```python
from build123d import *

# Parameters (mm, degrees)
SKETCH_1_W          = 180
SKETCH_1_H          = 50
EXTRUDE_1_DEPTH     = 30
SKETCH_2_W          = 40
SKETCH_2_H          = 50
EXTRUDE_2_DEPTH     = 80
FILLET_1_R          = 25
SKETCH_3_R          = 12.5
CUT_EXTRUDE_2_DEPTH = 145.913767462
SKETCH_7_W          = 25
SKETCH_7_H          = 50
EXTRUDE_5_DEPTH     = 80
EXTRUDE_6_REACH     = 213.019
SKETCH_9_W          = 25.5
SKETCH_9_H          = 50
CUT_EXTRUDE_3_DEPTH = 401.320460854
SKETCH_10_W         = 65
SKETCH_10_H         = 50
EXTRUDE_7_DEPTH     = 80
SKETCH_11_W         = 50
SKETCH_11_H         = 30
EXTRUDE_8_DEPTH     = 10
SKETCH_12_W         = 50
SKETCH_12_H         = 30
CUT_EXTRUDE_4_DEPTH = 5
SKETCH_13_R         = 7.5
CUT_EXTRUDE_5_DEPTH = 412.96204223


with BuildPart() as part:
    # Sketch 1 → Extrude 1 (new body)
    with BuildSketch(Plane(origin=(0, 0, 0), x_dir=(1, 0, 0), z_dir=(0, 1, 0))):
        with Locations((90, -25)):
            Rectangle(SKETCH_1_W, SKETCH_1_H)
    extrude(amount=EXTRUDE_1_DEPTH)

    # Sketch 2 → Extrude 2 (add)
    with BuildSketch(Plane.XZ):
        with Locations((90, 25)):
            Rectangle(SKETCH_2_W, SKETCH_2_H)
    extrude(amount=EXTRUDE_2_DEPTH)

    # Fillet 1
    fillet_1_edges = [part.edges().sort_by_distance(p)[0] for p in [
        (90, -80, 50),
        (90, -80, 0),
    ]]
    fillet(fillet_1_edges, radius=FILLET_1_R - 0.0001)  # a hair under: the kernel refuses the full size

    # Sketch 3 → Cut-Extrude 2 (cut, through all)
    with BuildSketch(Plane(origin=(110, 0, 0), x_dir=(0, 0, -1), z_dir=(1, 0, 0))):
        with Locations((-25, -55)):
            Circle(SKETCH_3_R)
    extrude(amount=-CUT_EXTRUDE_2_DEPTH, mode=Mode.SUBTRACT)

    # Sketch 7 → Extrude 5 (add)
    with BuildSketch(Plane(origin=(0, 30, 0), x_dir=(1, 0, 0), z_dir=(0, 1, 0))):
        with Locations((19.5, -25)):
            Rectangle(SKETCH_7_W, SKETCH_7_H)
        with Locations((160.5, -25)):
            Rectangle(SKETCH_7_W, SKETCH_7_H)
    extrude(amount=EXTRUDE_5_DEPTH)

    # Extrude 6: up to this face of the body (flat: up to its plane)
    extrude_6_end = Plane(part.part.faces().sort_by_distance((7, 70, 25))[0])
    # Sketch 8 → Extrude 6 (add, up to the picked face)
    with BuildSketch(Plane(origin=(173, 0, 0), x_dir=(0, 0, -1), z_dir=(1, 0, 0)), mode=Mode.PRIVATE) as extrude_6_sk1:
        with BuildLine():
            Line((0, 110), (-79.29372145, 110))
            add(Edge.make_bspline(
                [(-79.29372145, 110), (123.322725029, 174.375095478), (335.808448859, 110)],
                knots=[0, 0, 0, 1, 1, 1], degree=2))
            add(Edge.make_bspline(
                [(335.808448859, 110), (344.655163531, 85.008885119), (332.386652106, 65.024574676)],
                knots=[0, 0, 0, 1, 1, 1], degree=2))
            add(Edge.make_bspline(
                [(332.386652106, 65.024574676), (334.882025134, 94.793074398), (307.328252939, 102.88474179)],
                knots=[0, 0, 0, 1, 1, 1], degree=2))
            add(Edge.make_bspline(
                [(307.328252939, 102.88474179), (153.571097441, 138.708355764), (0, 110)],
                knots=[0, 0, 0, 1, 1, 1], degree=2))
        make_face()
    extrude_6_tool1 = split(extrude(extrude_6_sk1.sketch, amount=-EXTRUDE_6_REACH, mode=Mode.PRIVATE), bisect_by=extrude_6_end, keep=Keep.BOTH, mode=Mode.PRIVATE)
    add(extrude_6_tool1.solids().sort_by(Axis((173, 122.914419, -143.709252), (-1, 0, 0)))[0])

    # Sketch 9 → Cut-Extrude 3 (cut, through all)
    with BuildSketch(Plane(origin=(0, 30, 0), x_dir=(1, 0, 0), z_dir=(0, 1, 0))):
        Polygon((57.5, -50), (32, -50), (32, 0), (57.5, 0), (57.5, 350.332715619), (7, 350.332715619), (7, -79.29372145), (57.5, -79.29372145), align=None)
        Polygon((148, -50), (122.5, -50), (122.5, -79.29372145), (173, -79.29372145), (173, 350.332715619), (122.5, 350.332715619), (122.5, 0), (148, 0), align=None)
        with Locations((44.75, -25)):
            Rectangle(SKETCH_9_W, SKETCH_9_H)
        with Locations((135.25, -25)):
            Rectangle(SKETCH_9_W, SKETCH_9_H)
    extrude(amount=CUT_EXTRUDE_3_DEPTH, mode=Mode.SUBTRACT)


with BuildPart() as cut_extrude_3_piece_1:
    # of the separate pieces the step leaves, piece 1, a body of its own (cut_extrude_3_pieces)
    add(part.part.solids().sort_by_distance((122.5, 110, 0))[0])



with BuildPart() as cut_extrude_3_piece_2:
    # of the separate pieces the step leaves, piece 2, a body of its own (cut_extrude_3_pieces)
    add(part.part.solids().sort_by_distance((110, -55.0001, 0))[0])


with BuildPart() as cut_extrude_3_piece_1_1:
    add(cut_extrude_3_piece_1.part)

    add(cut_extrude_3_piece_2.part)  # Extrude 7 merges Cut-Extrude 3 piece 2
    # Sketch 10 → Extrude 7 (add)
    with BuildSketch(Plane.XZ.offset(-110)):
        with Locations((90, 25)):
            Rectangle(SKETCH_10_W, SKETCH_10_H)
    extrude(amount=EXTRUDE_7_DEPTH)

    # Sketch 11 → Extrude 8 (add)
    with BuildSketch(Plane.ZY):
        with Locations((25, 15)):
            Rectangle(SKETCH_11_W, SKETCH_11_H)
    extrude(amount=EXTRUDE_8_DEPTH)

    # Sketch 12 → Cut-Extrude 4 (cut)
    with BuildSketch(Plane.ZY.offset(10)):
        with Locations((25, 15)):
            Rectangle(SKETCH_12_W, SKETCH_12_H)
    extrude(amount=-CUT_EXTRUDE_4_DEPTH, mode=Mode.SUBTRACT)

    # Sketch 13 → Cut-Extrude 5 (cut, through all)
    with BuildSketch(Plane.ZY.offset(5)):
        with Locations((25, 15)):
            Circle(SKETCH_13_R)
    extrude(amount=-CUT_EXTRUDE_5_DEPTH, mode=Mode.SUBTRACT)


solid = cut_extrude_3_piece_1_1.part
```
CAD build for the part. Positions are in the model's coordinates, mm. A direction names the side the tool comes from. Round coordinates to 2 decimals unless told otherwise and drop trailing zeros. Order: outer loops, then holes, each group sorted by start corner. A loop starts at its lowest first (then second) coordinate and runs counter-clockwise, first axis right, second up.
Item 1: Mould opens along Z. For faces 5 (the face through (151, 30, 25)), 6 (the face through (89, 26, 0)), 7 (the face through (89, 26, 50)) say: pulls with the +Z half, pulls with the -Z half, needs draft (parallel to the pull), parting line crosses it, or undercut.
Item 2: Saw through at C-C on y = -62. Write the cut outline in (x, z).
Item 3: Pin check, flat tip, straight feed: pin 1 (8 mm diameter, centred on x = 56.5, y = 35, fed in from +Z). Stop position of the tip, or through.
Item 4: Tool access for faces 1 (the face through (27, 30, 25)), 2 (the face through (122.5, 124, -85)), 3 (the face through (70, -31, 25)), 4 (the face through (145, 0, 25)): list every direction of +Z, -Z, +X, -X, +Y, -Y with a clear straight run to the whole face (end or side of a thin tool).
Item 5: Saw through at B-B on x = 6.5. Write the cut outline in (y, z).
Item 6: Probe line 1 along Y through (x, z) = (100.5, 25); line 2 along Y through (x, z) = (48, 25); line 3 along Z through (x, y) = (143, 18). List the from-to ranges inside material, lowest first.
Item 7: Saw through at A-A on y = 15. Write the cut outline in (x, z), then the cut area to 4 significant figures.
Item 8: Saw through at D-D on y = -35.5. Write the cut outline in (x, z), then the cut area to 3 significant figures.
Reported:
1. face 5: needs draft
1. face 6: undercut
1. face 7: pulls with the +Z half
2. outline: (70, 1) - (110, 1) - (110, 14.64) - (70, 14.64) - close; (70, 35.36) - (110, 35.36) - (110, 49) - (70, 49) - close
3. pin 1: stops at z = 50
4. face 1: +Z, -Z, -X, +Y
4. face 2: +Z, -Z, +X, +Y
4. face 3: +Z, -Z, -X, -Y
4. face 4: +Z, -Z, +X, -Y
5. outline: (0, 0) - (30, 0) - (30, 50) - (0, 50) - close; hole circle Ø15 at (15, 25)
6. line 1: y = -80 to -67.5, -42.5 to 7.5, 22.5 to 124.9
6. line 2: y = 0 to 7.5, 22.5 to 30
6. line 3: z = 0 to 18.13, 31.87 to 50
7. outline: (-5, 0) - (180, 0) - (180, 17.5) - (-5, 17.5) - close; (-5, 32.5) - (180, 32.5) - (180, 50) - (-5, 50) - close
7. area: 6,475 mm2
8. outline: (70, 0) - (110, 0) - (110, 50) - (70, 50) - close
8. area: 2,000 mm2
